Design review of the part built by this model. Coordinates are the model's own, in mm. Face numbers are marked on the shaded views. A direction names the side the tool comes from. Coordinates: 2 decimals unless noted, no trailing zeros. Loops run counter-clockwise (first coordinate to the right, second up) from the corner with the lowest first, then second, coordinate; pieces in that order, holes last. Notation, with made-up numbers: M 18.25,46.5 L 32.25,46.5 A29 cw 32.25,77.5 Z; hole C 50.25,76 d6. An arc over 180 degrees is marked long. Write item = value, one per line. Start each with the question number.
Autodesk Inventor part; units mm, degrees
ref_plane "YZ Plane" through (0, 0, 0) normal (1, 0, 0) x (0, 1, 0)
ref_plane "XZ Plane" through (0, 0, 0) normal (0, 1, 0) x (-1, 0, 0)
ref_plane "XY Plane" through (0, 0, 0) normal (0, 0, 1) x (1, 0, 0)
sketch "Sketch1" plane through (0, 0, 0) normal (1, 0, 0) x (0, 1, 0)
  line L0 (0, 0) -> (-152.4, 0)
  line L1 (-152.4, 0) -> (-152.4, -12.7)
  line L2 (-152.4, -12.7) -> (0, -12.7)
  line L3 (0, -12.7) -> (0, 0)
  line L4 (0, -12.7) -> (-12.7, -12.7)
  line L5 (-12.7, -63.5) -> (0, -63.5)
  line L6 (0, -63.5) -> (-152.4, -63.5)
  line L7 (-152.4, -63.5) -> (-152.4, -76.2)
  line L8 (-152.4, -76.2) -> (0, -76.2)
  line L9 (0, -76.2) -> (0, -63.5)
  line L10 (-152.4, 0) -> (-139.7, 0)
  line L11 (-139.7, 0) -> (-139.7, -76.2)
  line L12 (-139.7, -76.2) -> (-152.4, -76.2)
  line L13 (-152.4, -76.2) -> (-152.4, 0)
  dimension "d1" = 12.7
  dimension "d4" = 12.7
  dimension "d63" = 12.7
  dimension "d64" = 152.4
  dimension "d65" = 152.4
  dimension "d66" = 50.8
extrude "Extrusion1" add sketch "Sketch1" along normal blind 25.4
sketch "Sketch2" plane through (0, -152.4, -76.2) normal (0, 0, -1) x (-1, 0, 0)
  line L0 (0, 152.4) -> (-25.4, 152.4)
  line L1 (-25.4, 0) -> (-25.4, 152.4)
  point P0 (-12.7, 107.95)
  dimension "d8" = 44.45
  dimension "d9" = 25.4
  dimension "d10" = 12.7
hole "Hole1" at (12.7, -44.45, -76.2) direction (0, 0, 1) diameter 12.7 end through all
sketch "Sketch3" plane through (0, -152.4, -76.2) normal (0, 0, -1) x (-1, 0, 0)
  circle A0 centre (-12.7, 107.95) radius 6.35
  line L0 (0, 0) -> (0, 152.4)
  line L1 (0, 152.4) -> (-25.4, 152.4)
  line L2 (-25.4, 0) -> (-25.4, 152.4)
  line L3 (0, 0) -> (-25.4, 0)
  point P0 (-12.7, 50.8)
  dimension "d18" = 25.4
  dimension "d19" = 12.7
  dimension "d20" = 50.8
hole "Hole2" at (12.7, -101.6, -76.2) direction (0, 0, 1) diameter 18.4912 end through all
sketch "Sketch4" plane through (0, -152.4, -76.2) normal (0, 0, -1) x (-1, 0, 0)
  circle A0 centre (-12.7, 50.8) radius 9.2456
  circle A1 centre (-12.7, 107.95) radius 6.35
  line L0 (0, 0) -> (0, 152.4)
  line L1 (0, 152.4) -> (-25.4, 152.4)
  line L2 (-25.4, 0) -> (-25.4, 152.4)
  line L3 (0, 0) -> (-25.4, 0)
  point P0 (-5.6896, 26.797)
  point P1 (-5.6896, 74.803)
  dimension "d28" = 48.006
  dimension "d29" = 7.0104
  dimension "d30" = 7.0104
  dimension "d31" = 24.003
hole "Hole3" at (5.6896, -125.603, -76.2) at (5.6896, -77.597, -76.2) direction (0, 0, 1) diameter 3.7084 end through all
sketch "Sketch5" plane through (25.4, 0, 0) normal (1, 0, 0) x (0, 0, -1)
  line L0 (0, 0) -> (12.7, 0)
  line L1 (12.7, 0) -> (12.7, -25.4)
  line L2 (12.7, -25.4) -> (0, -25.4)
  line L3 (0, -25.4) -> (0, 0)
  line L4 (0, 0) -> (0, -152.4)
  line L5 (12.7, 0) -> (0, 0)
  dimension "d39" = 12.7
  dimension "d67" = 25.4
  dimension "d68" = 0
  dimension "d69" = 0
extrude "Extrusion2" add sketch "Sketch5" along normal blind 127
sketch "Sketch8" plane through (0, -139.7, -12.7) normal (0, 0, -1) x (-1, 0, 0)
  line L0 (-152.4, 114.3) -> (-152.4, 139.7)
  line L1 (0, 139.7) -> (-152.4, 139.7)
  point P0 (-133.35, 127)
  dimension "d70" = 19.05
  dimension "d71" = 25.4
  dimension "d72" = 12.7
hole "Hole6" at (133.35, -12.7, -12.7) direction (0, 0, 1) diameter 12.7 end through all
equation "\"d4\" = d1"
equation "\"d65\" = d64"
properties part number "shooter" material "Aluminum 6061"
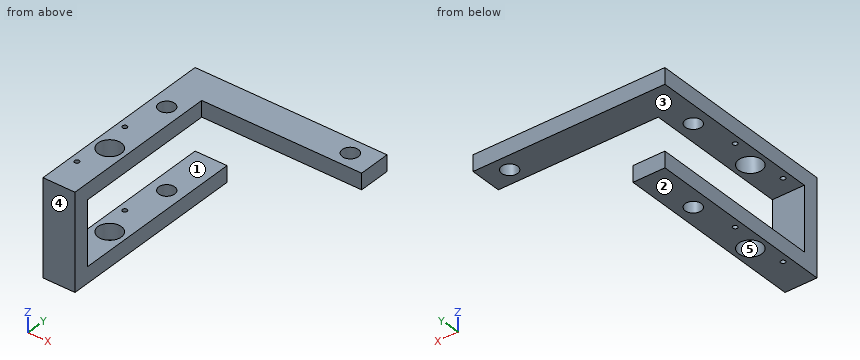
Q1. Add section B-B on x = 12.7. State the section outline as (y, z) points, plus the area to 3 significant figures.
Q2. Add section A-A on y = -44.45. State the section outline as (x, z) points.
Q3. Mouldability with a two-part tool opening along Y and no side actions: class the marked faces 3, 4 and 5 as released by +Y, released by -Y, zero draft, split by the parting line, or undercut.
Q4. For the marked faces 1 and 2, list the 3-axis set-ups (+Z, -Z, +X, -X, +Y, -Y) from which the entire face can be reached by the end or side of a thin tool; tool diameter is ignored.
Q5. Add section C-C on y = -12.7. State the section outline as (x, z) points.
Q6. Add section D-D on x = 133.35. State the section outline as (y, z) points.
Q7. To check wall thickness, follow line 1 (Y direction, x = 12.7, z = -70); line 2 (Z direction, x = 12.5, y = -121); line 3 (X direction, y = -102.5, z = -72.5). State the ranges of each line that lie inside material, in increasing order. Write a range as from..to.
Q8. Clearance check with flat-ended pins moving along their axes: P1, Ø10, axis at y = -18.5, z = -66.5, coming from the +X side; P2, Ø20.5, axis at x = 14, z = -40, coming from the +Y side; P3, Ø14, axis at x = 114.5, z = -6, coming from the -Y side. State where each tip first meets the part, or that it passes through.
Values follow:
q1.outline = M -152.4,-76.2 L -110.85,-76.2 L -110.85,-63.5 L -139.7,-63.5 L -139.7,-12.7 L -110.85,-12.7 L -110.85,0 L -152.4,0 Z; M -92.35,-76.2 L -50.8,-76.2 L -50.8,-63.5 L -92.35,-63.5 Z; M -92.35,-12.7 L -50.8,-12.7 L -50.8,0 L -92.35,0 Z; M -38.1,-76.2 L 0,-76.2 L 0,-63.5 L -38.1,-63.5 Z; M -38.1,-12.7 L 0,-12.7 L 0,0 L -38.1,0 Z
q1.area = 3,720 mm2
q2.outline = M 0,-76.2 L 6.35,-76.2 L 6.35,-63.5 L 0,-63.5 Z; M 0,-12.7 L 6.35,-12.7 L 6.35,0 L 0,0 Z; M 19.05,-76.2 L 25.4,-76.2 L 25.4,-63.5 L 19.05,-63.5 Z; M 19.05,-12.7 L 25.4,-12.7 L 25.4,0 L 19.05,0 Z
q3.face_3 = zero draft
q3.face_4 = released by -Y
q3.face_5 = undercut
q4.face_1 = +X, -X, +Y
q4.face_2 = -Z, +X, -X, +Y, -Y
q5.outline = M 0,-76.2 L 25.4,-76.2 L 25.4,-63.5 L 0,-63.5 Z; M 0,-12.7 L 127,-12.7 L 127,0 L 0,0 Z; M 139.7,-12.7 L 152.4,-12.7 L 152.4,0 L 139.7,0 Z
q6.outline = M -25.4,-12.7 L -19.05,-12.7 L -19.05,0 L -25.4,0 Z; M -6.35,-12.7 L 0,-12.7 L 0,0 L -6.35,0 Z
q7.line_1 = -152.4..-110.85, -92.35..-50.8, -38.1..0
q7.line_2 = -76.2..-63.5, -12.7..0
q7.line_3 = 0..3.5, 21.9..25.4
q8.P1 = 25.4
q8.P2 = -139.7
q8.P3 = -25.4
